Work out the finished part from the listing and answer in its coordinate system (mm). A direction names the side the tool comes from. Give positions to 0.01 mm unless a question says otherwise; leave off trailing zeros. Loops run counter-clockwise (first coordinate to the right, second up) from the corner with the lowest first, then second, coordinate; pieces in that order, holes last.
```python
from build123d import *

# Parameters (mm, degrees)
BOSS_EXTRUDE1_DEPTH = 16.8656
CHAMFER1_SIZE       = 0.254
SKETCH3_R           = 1.5875
CUT_EXTRUDE1_DEPTH  = 16.3576
SKETCH4_R           = 2.286
CUT_EXTRUDE2_DEPTH  = 17.8656


with BuildPart() as part:
    # Sketch1 → Boss-Extrude1 (new body)
    with BuildSketch(Plane(origin=(0, 0, 0), x_dir=(1, 0, 0), z_dir=(0, 1, 0))):
        with BuildLine():
            Line((0, 13.97), (25.4, 13.97))
            ThreePointArc((25.4, 13.97), (39.37, 0), (25.4, -13.97))
            Line((25.4, -13.97), (0, -13.97))
            ThreePointArc((0, -13.97), (-13.97, 0), (0, 13.97))
        make_face()
    extrude(amount=BOSS_EXTRUDE1_DEPTH)

    # Chamfer1
    chamfer1_edges = [part.edges().sort_by_distance(p)[0] for p in [
        (39.37, 16.8656, 0),
        (12.7, 16.8656, -13.97),
        (-13.97, 16.8656, 0),
        (12.7, 16.8656, 13.97),
    ]]
    chamfer(chamfer1_edges, length=CHAMFER1_SIZE)

    # Sketch3 → Cut-Extrude1 (cut)
    with BuildSketch(Plane(origin=(0, 16.8656, 0), x_dir=(1, 0, 0), z_dir=(0, 1, 0))):
        with Locations((25.4, 6.096)):
            Circle(SKETCH3_R)
        with Locations((31.496, 0)):
            Circle(SKETCH3_R)
        with Locations((25.4, -6.096)):
            Circle(SKETCH3_R)
        with Locations((19.304, 0)):
            Circle(SKETCH3_R)
        with Locations((-6.096, 0)):
            Circle(SKETCH3_R)
        with Locations((6.096, 0)):
            Circle(SKETCH3_R)
        with Locations((0, -6.096)):
            Circle(SKETCH3_R)
        with Locations((0, 6.096)):
            Circle(SKETCH3_R)
    extrude(amount=-CUT_EXTRUDE1_DEPTH, mode=Mode.SUBTRACT)

    # Sketch4 → Cut-Extrude2 (cut, through all)
    with BuildSketch(Plane(origin=(0, 16.8656, 0), x_dir=(1, 0, 0), z_dir=(0, 1, 0))):
        with Locations((12.7, 10.16)):
            Circle(SKETCH4_R)
        with Locations((12.7, -10.16)):
            Circle(SKETCH4_R)
    extrude(amount=-CUT_EXTRUDE2_DEPTH, mode=Mode.SUBTRACT)


solid = part.part
```
Q1. Given pin 1 (1.6 mm diameter, centred on x = 25, z = -6.5, fed in from +Y); pin 2 (6 mm diameter, centred on y = 7.5, z = 5, fed in from +X); pin 3 (4 mm diameter, centred on y = 4.5, z = -9.5, fed in from -X), each flat-ended and moving along its own axis, determine where each tip first touches the part or whether it passes through.
Q2. Consider line 1 along X through (y, z) = (6, 0); line 2 along Z through (x, y) = (0, 12.5); line 3 along Z through (x, y) = (12.7, 5.75). Determine where each line is inside the solid, lowest interval first.
Q3. Which of the six approach directions +Z, -Z, +X, -X, +Y, -Y give full straight-line access (tool end or side, diameter ignored) to faces 1 (the face through (13.75, 8.55, 12.19)), 2 (the face through (4.51, 8.8, -0.07))?
Q4. Section B-B on z = 0 is taken. Give the vertices of the cut face in (x, y).
Q5. Section A-A on x = 12.7 is taken. Give the vertices of the cut face in (y, z).
Q6. Section C-C on y = 12 is taken. State how many separate pieces and enclosed holes the cut face has, plus the area to 3 significant figures.
Check result:
1. pin 1: stops at y = 0.51
1. pin 2: stops at x = 39.23
1. pin 3: stops at x = -11.79
2. line 1: x = -13.97 to -7.68, -4.51 to 4.51, 7.68 to 17.72, 20.89 to 29.91, 33.08 to 39.37
2. line 2: z = -13.97 to -7.68, -4.51 to 4.51, 7.68 to 13.97
2. line 3: z = -13.97 to -12.45, -7.87 to 7.87, 12.45 to 13.97
3. face 1: +Y, -Y
3. face 2: +Y
4. outline: (-13.97, 0) - (39.37, 0) - (39.37, 16.61) - (39.12, 16.87) - (33.08, 16.87) - (33.08, 0.51) - (29.91, 0.51) - (29.91, 16.87) - (20.89, 16.87) - (20.89, 0.51) - (17.72, 0.51) - (17.72, 16.87) - (7.68, 16.87) - (7.68, 0.51) - (4.51, 0.51) - (4.51, 16.87) - (-4.51, 16.87) - (-4.51, 0.51) - (-7.68, 0.51) - (-7.68, 16.87) - (-13.72, 16.87) - (-13.97, 16.61) - close
5. outline: (0, -13.97) - (16.61, -13.97) - (16.87, -13.72) - (16.87, -12.45) - (0, -12.45) - close; (0, -7.87) - (16.87, -7.87) - (16.87, 7.87) - (0, 7.87) - close; (0, 12.45) - (16.87, 12.45) - (16.87, 13.72) - (16.61, 13.97) - (0, 13.97) - close
6. separate pieces: 1
6. enclosed holes: 10
6. area: 1,230 mm2
